Geometry: see drawing. Coordinates: mm, zero at the bounding-box minimum. Give positions to 0.01 mm unless a question says otherwise; leave off trailing zeros. Loops run counter-clockwise (first coordinate to the right, second up) from the corner with the lowest first, then second, coordinate; pieces in that order, holes last. Notation, with made-up numbers: M 67.25,-8.75 L 82.25,-8.75 A31 ccw 82.25,19.25 Z; hole C 85,25 d6. An arc over 180 degrees is marked long. Put each result on its own line as item: value.
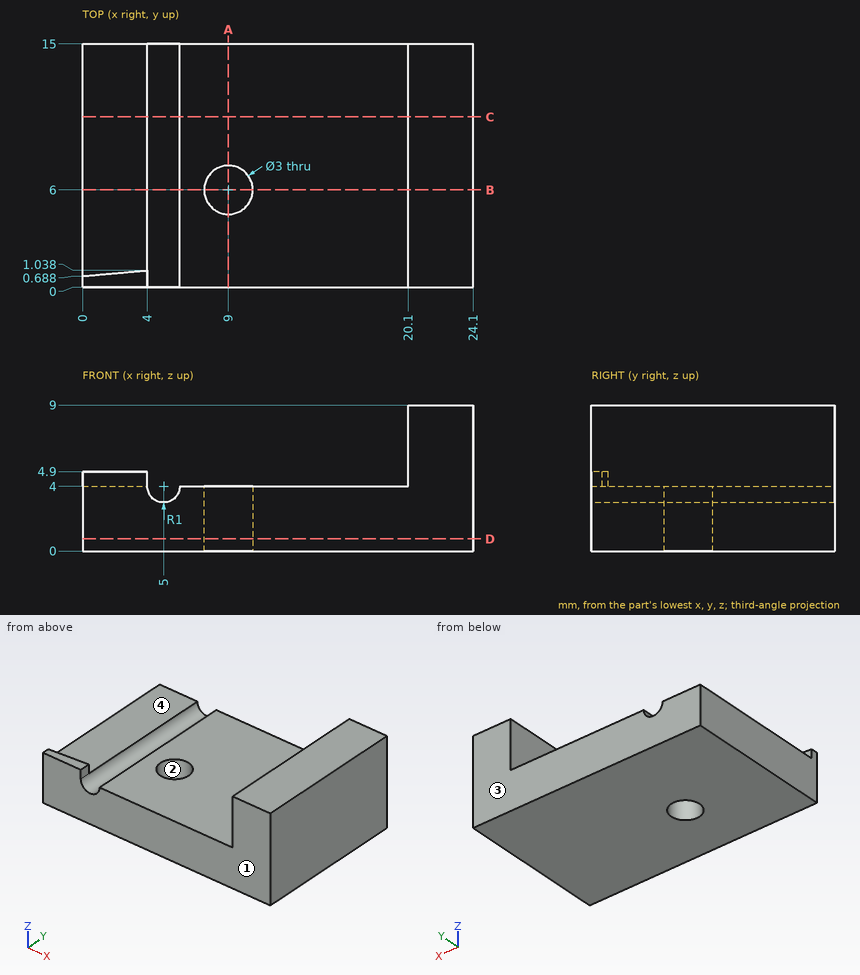
Item 1: Mould query, pull axis Y, two halves, no side actions, for the marked faces 1, 2, 3 and 4. Classes: pulls with the +Y half, pulls with the -Y half, needs draft (parallel to the pull), parting line crosses it, or undercut.
Output values:
face 1: pulls with the -Y half
face 2: undercut
face 3: pulls with the +Y half
face 4: needs draft
Item 2: Section A-A on x = 9. Output: boundary loops of the cut face in (y, z), then the cut area to 3 significant figures.
Output values:
outline: M 0,0 L 4.5,0 L 4.5,4 L 0,4 Z; M 7.5,0 L 15,0 L 15,4 L 7.5,4 Z
area: 48.0 mm²
Item 3: Line query: probe 1 along Y at (x, z) = (9, 1.55); probe 2 along Z at (x, y) = (12.5, 4.25); probe 3 along X at (y, z) = (7, 7). Output: solid intervals per line, ascending. Write a range as [from, to].
Output values:
probe 1: [0, 4.5], [7.5, 15]
probe 2: [0, 4]
probe 3: [20.1, 24.1]
Item 4: Pin query (flat end, axial travel): pin 1 Ø3 at (x, y) = (1, 10) entering from +Z; pin 2 Ø0.8 at (x, y) = (2.5, 0.5) entering from +Z; pin 3 Ø4 at (y, z) = (4.5, 6.5) entering from -X. Return the tip coordinate at first contact, or that it passes through.
Output values:
pin 1: z = 4
pin 2: z = 4.9
pin 3: x = 20.1
Item 5: Section B-B on y = 6. Output: boundary loops of the cut face in (x, z), then the cut area to 3 significant figures.
Output values:
outline: M 0,0 L 7.5,0 L 7.5,4 L 6,4 A1 cw 4,4 L 0,4 Z; M 10.5,0 L 24.1,0 L 24.1,9 L 20.1,9 L 20.1,4 L 10.5,4 Z
area: 103 mm²
Item 6: Section D-D on z = 0.75. Output: boundary loops of the cut face in (x, y), then the cut area to 3 significant figures.
Output values:
outline: M 0,0 L 24.1,0 L 24.1,15 L 0,15 Z; hole C 9,6 d3
area: 354 mm²
Item 7: Section C-C on y = 10.5. Output: boundary loops of the cut face in (x, z).
Output values:
outline: M 0,0 L 24.1,0 L 24.1,9 L 20.1,9 L 20.1,4 L 6,4 A1 cw 4,4 L 0,4 Z
